The listing builds one solid part. Answer for the finished solid, in the listing's coordinates (mm). Coordinates: 2 decimals unless noted, no trailing zeros. Write each loop counter-clockwise with the first axis right and the second up, starting at its lowest first coordinate (ties: lowest second). Pieces come first, ordered by that corner, then holes. Notation, with made-up numbers: M 48,59 L 91,59 A26 ccw 91,92 Z; hole C -12,54.25 d7. An arc over 180 degrees is marked long. Answer as a JSON object with one key per item and string values. Group by question number.
from build123d import *

# Parameters (mm, degrees)
BOSS_EXTRUDE1_DEPTH = 10
CUT_EXTRUDE1_DEPTH  = 10
SKETCH4_RX          = 87.174762469
SKETCH4_RY          = 66.453525419
CUT_EXTRUDE2_DEPTH  = 10
SKETCH5_W           = 26.438615702
SKETCH5_H           = 10
CUT_EXTRUDE5_DEPTH  = 30
SKETCH6_W           = 22.623740515
SKETCH6_H           = 10
CUT_EXTRUDE6_DEPTH  = 10


with BuildPart() as part:
    # Sketch1 → Boss-Extrude1 (new body)
    with BuildSketch(Plane.XY):
        with BuildLine():
            Line((-427.107921319, -118.031926349), (-575.271952131, -118.031926349))
            Line((-575.271952131, -118.031926349), (-575.271952131, -158.031926349))
            Line((-575.271952131, -158.031926349), (-192.080048862, -158.031926349))
            Line((-192.080048862, -158.031926349), (-192.080048862, -148.031926349))
            add(Edge.make_bspline(
                [(-192.080048862, -148.031926349), (-157.837008984, -114.51884489), (-75.168475425, -70.609825384), (16.241097891, -49.938935327), (61.818541816, -59.568417069)],
                knots=[0, 0, 0, 0, 0.513639289, 1, 1, 1, 1], degree=3))
            Line((61.818541816, -59.568417069), (50.930294818, 169.898138867))
            Line((50.930294818, 169.898138867), (34.940241092, 184.040274491))
            Line((34.940241092, 184.040274491), (-18.862584596, 136.455265033))
            Line((-18.862584596, 136.455265033), (-2.872530869, 122.313129409))
            Line((-2.872530869, 122.313129409), (-49.270535503, 81.277190105))
            add(Edge.make_bspline(
                [(-427.107921319, -118.031926349), (-356.64028899, -119.331018895), (-244.870528992, -125.219604065), (-108.651854921, -44.255191333), (-41.057154586, 17.202634848), (-49.270535503, 81.277190105)],
                knots=[0, 0, 0, 0, 0.468078311, 0.64359283, 1, 1, 1, 1], degree=3))
        make_face()
    extrude(amount=BOSS_EXTRUDE1_DEPTH)

    # Sketch2 → Cut-Extrude1 (cut, symmetric)
    with BuildSketch(Plane(origin=(28.004521107, -27.258908823, 34.059132337), x_dir=(0.8415259589150524, 0.33755828909978275, -0.4217682561930533), z_dir=(0.5402166791872512, -0.5258335661753164, 0.6570121766080502))):
        Polygon((55.096893941, -25.281928608), (25.403338602, -49.506612522), (-27.145369489, -41.573178566), (2.888217841, -17.531746483), (44.92299541, 24.503031085), (95.182381766, 9.000336469), align=None)
    extrude(amount=CUT_EXTRUDE1_DEPTH, both=True, mode=Mode.SUBTRACT)


with BuildPart() as cut_extrude1_kept_piece:
    # of the separate pieces the step leaves, the one the design keeps (cut_extrude1_pieces_kept)
    add(part.part.solids().sort_by_distance((-427.107921319, -118.031926349, 0))[0])

    # Sketch4 → Cut-Extrude2 (cut)
    with BuildSketch(Plane.XY.offset(10)):
        with Locations(Location((76.445934185, 53.167488188), (0, 0, -90))):
            Ellipse(SKETCH4_RX, SKETCH4_RY)
    extrude(amount=-CUT_EXTRUDE2_DEPTH, mode=Mode.SUBTRACT)

    # Sketch5 → Cut-Extrude5 (cut)
    with BuildSketch(Plane(origin=(-379.077692484, 0, -259.207509724), x_dir=(0.5644444444444446, 0, -0.8254710589328995), z_dir=(0.8254710589328994, 0, 0.5644444444444445))):
        with Locations((-327.230934206, -123.031926349)):
            Rectangle(SKETCH5_W, SKETCH5_H)
        with Locations((-327.230934206, -143.031926349)):
            Rectangle(SKETCH5_W, SKETCH5_H)
    extrude(amount=-CUT_EXTRUDE5_DEPTH, mode=Mode.SUBTRACT)

    # Sketch6 → Cut-Extrude6 (cut)
    with BuildSketch(Plane.XZ.offset(158.031926349)):
        with Locations((-203.39191912, 5)):
            Rectangle(SKETCH6_W, SKETCH6_H)
    extrude(amount=-CUT_EXTRUDE6_DEPTH, mode=Mode.SUBTRACT)


solid = cut_extrude1_kept_piece.part
Item 1: Consider L1, parallel to Y at x = -506.5, z = 6; L2, parallel to Y at x = -323, z = 6.25; L3, parallel to X at y = 165, z = 4.5. Determine where each line is inside the solid, lowest interval first. Write a range as from..to.
Item 2: Flat-ended cylindrical pins translate along their axes: pin 1 Ø3 at (x, z) = (-199, 6.5) entering from -Y; pin 2 Ø3 at (x, z) = (-488.5, 5) entering from +Y; pin 3 Ø6 at (y, z) = (-9.5, 2) entering from +X. Find the tip coordinate at first contact, or state that the pin passes through.
Item 3: A cutting plane is placed at B-B, the plane y = 161. Write down the section's boundary in (x, z), and give its area (3 significant figures).
Item 4: For a pull along Y with two mould halves and no side action, classify faces 1 (the face through (8.415, 160.581, 4.93)), 2 (the face through (-11, 129.5, 4.9)), 3 (the face through (-170, -88, 10)), 4 (the face through (-25.75, 102.08, 4.93)) as +Y half, -Y half, draft (parallel to the pull), parting line (faces both ways), or undercut.
Item 5: A cutting plane is placed at A-A, the plane x = -537. Write down the section's boundary in (y, z), and give its area (3 significant figures).
Answer:
{
 "1": {"L1": "-158.03..-118.03", "L2": "-158.03..-118.35", "L3": "13.41..51.16"},
 "2": {"pin 1": "y = -148.03", "pin 2": "y = -118.03", "pin 3": "x = 32.74"},
 "3": {"outline": "M 8.89,0 L 51.35,0 L 51.35,10 L 8.89,10 Z", "area": "425 mm2"},
 "4": {"face 1": "+Y half", "face 2": "undercut", "face 3": "draft", "face 4": "undercut"},
 "5": {"outline": "M -158.03,0 L -118.03,0 L -118.03,10 L -158.03,10 Z", "area": "400 mm2"}
}
